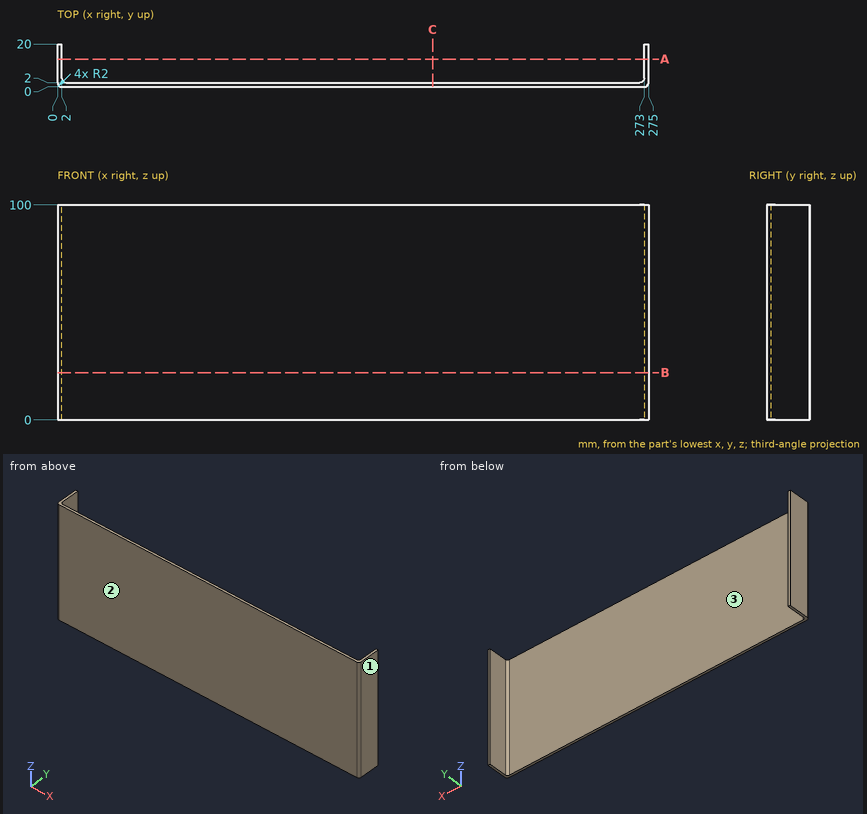
For this review, use the dimensioned drawing (mm, ordinates from the lowest corner) and the shaded views. Round coordinates to 2 decimals unless told otherwise and drop trailing zeros. Write each loop counter-clockwise with the first axis right and the second up, starting at its lowest first coordinate (ties: lowest second). Pieces come first, ordered by that corner, then holes. Notation, with made-up numbers: (48.5, 37.25) - (86.5, 37.25) arc R16 cw to (86.5, 51.25) - close; hole circle Ø1 at (-31.75, 80.25). An arc over 180 degrees is marked (long way). Answer as CSV lines item,"result". Start each with the question number.
(1) Draft analysis for pull direction X (two halves, no side actions). For the marked faces 1, 2 and 3, state which applies: pulls with the +X half, pulls with the -X half, needs draft (parallel to the pull), parting line crosses it, or undercut.
(2) We need section C-C on x = 174.5. State the section outline as (y, z) points.
(3) To check wall thickness, follow line 1 (X direction, y = 10.5, z = 41); line 2 (Y direction, x = 28.5, z = 35.5); line 3 (X direction, y = 2.75, z = 13). State the ranges of each line that lie inside material, in increasing order.
(4) We need section B-B on z = 22. State the section outline as (x, y) points, plus the area to 3 significant figures.
(5) We need section A-A on y = 13. State the section outline as (x, z) points.
(6) For pin 1 Ø10 at (x, z) = (123, 42) entering from +Y, flat-tipped, find the tip position at first contact; note if it passes through.
Worked answers:
1,face 1,"pulls with the +X half"
1,face 2,"needs draft"
1,face 3,"undercut"
2,outline,"(0, 0) - (2, 0) - (2, 100) - (0, 100) - close"
3,line 1,"0 to 2, 273 to 275"
3,line 2,"0 to 2"
3,line 3,"0 to 2.44, 272.56 to 275"
4,outline,"(0, 2) arc R2 ccw to (2, 0) - (273, 0) arc R2 ccw to (275, 2) - (275, 20) - (273, 20) - (273, 4) arc R2 cw to (271, 2) - (4, 2) arc R2 cw to (2, 4) - (2, 20) - (0, 20) - close"
4,area,"622 mm²"
5,outline,"(0, 0) - (2, 0) - (2, 100) - (0, 100) - close; (273, 0) - (275, 0) - (275, 100) - (273, 100) - close"
6,pin 1,"y = 2"
